```python
from build123d import *

# Parameters (mm, degrees)
BOSS_EXTRUDE2_DEPTH = 25
CUT_EXTRUDE1_REACH  = 76.865
SKETCH5_R           = 2.5
CUT_EXTRUDE4_DEPTH  = 51.520709


with BuildPart() as part:
    # Sketch2 → Boss-Extrude2 (new body)
    with BuildSketch(Plane(origin=(0, 0, 0), x_dir=(0, 0, -1), z_dir=(1, 0, 0))):
        with BuildLine():
            Line((0, 0), (59.16515139, 0))
            ThreePointArc((59.16515139, 0), (67.935731583, -14.803844614), (50.738650505, -15.384615385))
            ThreePointArc((50.738650505, -15.384615385), (49.651853624, -14.368825942), (48.21070024, -14))
            Line((48.21070024, -14), (45, -14))
            Line((45, -14), (0, -14))
            Line((0, -14), (0, -6.25))
            Line((0, -6.25), (47.230433128, -6.25))
            ThreePointArc((47.230433128, -6.25), (50.576761962, -7.534884479), (52.203232404, -10.729166667))
            ThreePointArc((52.203232404, -10.729166667), (65.645099511, -12.64769189), (54.705893308, -4.604166667))
            ThreePointArc((54.705893308, -4.604166667), (53.213216965, -5.454829079), (51.520708964, -5.75))
            Line((51.520708964, -5.75), (0, -5.75))
            Line((0, -5.75), (0, 0))
        make_face()
    extrude(amount=BOSS_EXTRUDE2_DEPTH)

    # Sketch5 → Cut-Extrude1 (cut, up to next)
    with BuildSketch(Plane.XZ.offset(14), mode=Mode.PRIVATE) as cut_extrude1_sk1:
        with Locations(Location((12.5, -30.56070024, 0), (0, 0, 270))):
            Circle(SKETCH5_R)
    cut_extrude1_tool1 = extrude(cut_extrude1_sk1.sketch, amount=-CUT_EXTRUDE1_REACH, mode=Mode.PRIVATE) & part.part
    # Sketch5 → Cut-Extrude1 (cut, up to next)
    with BuildSketch(Plane.XZ.offset(14), mode=Mode.PRIVATE) as cut_extrude1_sk2:
        with Locations(Location((12.5, -38.19070024, 0), (0, 0, 270))):
            Circle(SKETCH5_R)
    cut_extrude1_tool2 = extrude(cut_extrude1_sk2.sketch, amount=-CUT_EXTRUDE1_REACH, mode=Mode.PRIVATE) & part.part
    # Sketch5 → Cut-Extrude1 (cut, up to next)
    with BuildSketch(Plane.XZ.offset(14), mode=Mode.PRIVATE) as cut_extrude1_sk3:
        with Locations(Location((12.5, -44.84070024, 0), (0, 0, 270))):
            Circle(SKETCH5_R)
    cut_extrude1_tool3 = extrude(cut_extrude1_sk3.sketch, amount=-CUT_EXTRUDE1_REACH, mode=Mode.PRIVATE) & part.part
    add(cut_extrude1_tool1.solids().sort_by_distance((12.5, -14, -30.5607))[0], mode=Mode.SUBTRACT)
    add(cut_extrude1_tool2.solids().sort_by_distance((12.5, -14, -38.1907))[0], mode=Mode.SUBTRACT)
    add(cut_extrude1_tool3.solids().sort_by_distance((12.5, -14, -44.8407))[0], mode=Mode.SUBTRACT)

    # Sketch7 → Cut-Extrude4 (cut)
    with BuildSketch(Plane.XY):
        with BuildLine():
            Line((22.5, -6.25), (22.5, -5.75))
            ThreePointArc((22.5, -5.75), (12.5, -2), (2.5, -5.75))
            Line((2.5, -5.75), (2.5, -6.25))
            ThreePointArc((2.5, -6.25), (12.5, -10), (22.5, -6.25))
        make_face()
    extrude(amount=-CUT_EXTRUDE4_DEPTH, mode=Mode.SUBTRACT)


solid = part.part
```
Work out the finished part from the listing and answer in its coordinate system (mm). A direction names the side the tool comes from. Give positions to 0.01 mm unless a question says otherwise; leave off trailing zeros. Write each loop counter-clockwise with the first axis right and the second up, starting at its lowest first coordinate (ties: lowest second). Pieces come first, ordered by that corner, then holes.
(1) Which of the six approach directions +Z, -Z, +X, -X, +Y, -Y give full straight-line access (tool end or side, diameter ignored) to faces 5 (the cylindrical face through (12.325, -5.447, -53.236)), 6 (the cylindrical face through (10.979, -11.926, -42.857)), 7 (the flat face through (24, -6.25, -23)), 8 (the flat face through (12, -9, -51.521))?
Final values:
face 5: +X, -X
face 6: -Y
face 7: +Z, +X, -X
face 8: +Z
(2) The part is cut by section D-D on x = 17. Write down the section's boundary in (y, z).
Final values:
outline: (-15.38, -50.74) arc R10 ccw (long way) to (0, -59.17) - (0, 0) - (-2.68, 0) - (-2.68, -51.52) - (-5.75, -51.52) arc R5 ccw to (-4.6, -54.71) arc R7 cw (long way) to (-10.73, -52.2) arc R5 ccw to (-8.68, -51.52) - (-9.32, -51.52) - (-9.32, 0) - (-14, 0) - (-14, -48.21) arc R3 cw to start
(3) The part is cut by section A-A on z = -21. Write down the section's boundary in (x, y).
Final values:
outline: (0, -14) - (25, -14) - (25, -6.25) - (22.5, -6.25) arc R15.21 cw to (2.5, -6.25) - (0, -6.25) - close; (0, -5.75) - (2.5, -5.75) arc R15.21 cw to (22.5, -5.75) - (25, -5.75) - (25, 0) - (0, 0) - close
(4) The mould has two halves that part along Y. Classify faces 1 (the flat face through (12, -14, -24)), 2 (the cylindrical face through (12.32, -9.49, -51.91)), 3 (the flat face through (12.3, -1.6, 0)), 4 (the cylindrical face through (12.32, -14.55, -68.07)): pulls with the +Y half, pulls with the -Y half, needs draft (parallel to the pull), parting line crosses it, or undercut.
Final values:
face 1: pulls with the -Y half
face 2: undercut
face 3: needs draft
face 4: parting line crosses it
(5) Flat-ended cylindrical pins translate along their axes: pin 1 Ø1.2 at (x, z) = (23, -35) entering from -Y; pin 2 Ø8 at (x, y) = (7, -4) entering from -Z; pin 3 Ø1.5 at (x, y) = (7.5, -6.5) entering from -Z. Find the tip coordinate at first contact, or state that the pin passes through.
Final values:
pin 1: stops at y = -14
pin 2: stops at z = -68.96
pin 3: stops at z = -68.78
(6) The part is cut by section C-C on z = -45. Write down the section's boundary in (x, y), plus the area to 3 significant figures.
Final values:
outline: (0, -14) - (10.01, -14) - (10.01, -9.79) arc R15.21 cw to (2.5, -6.25) - (0, -6.25) - close; (0, -5.75) - (2.5, -5.75) arc R15.21 cw to (22.5, -5.75) - (25, -5.75) - (25, 0) - (0, 0) - close; (14.99, -14) - (25, -14) - (25, -6.25) - (22.5, -6.25) arc R15.21 cw to (14.99, -9.79) - close
area: 214 mm2
(7) The part is cut by section B-B on x = 12.5. Write down the section's boundary in (y, z), plus the area to 3 significant figures.
Final values:
outline: (-15.38, -50.74) arc R10 ccw (long way) to (0, -59.17) - (0, 0) - (-2, 0) - (-2, -51.52) - (-5.75, -51.52) arc R5 ccw to (-4.6, -54.71) arc R7 cw (long way) to (-10.73, -52.2) arc R5 ccw to (-8.68, -51.52) - (-10, -51.52) - (-10, -47.34) - (-14, -47.34) - (-14, -48.21) arc R3 cw to start; (-14, -42.34) - (-10, -42.34) - (-10, -40.69) - (-14, -40.69) - close; (-14, -35.69) - (-10, -35.69) - (-10, -33.06) - (-14, -33.06) - close; (-14, -28.06) - (-10, -28.06) - (-10, 0) - (-14, 0) - close
area: 395 mm2
(8) Straight lines are drawn through the part: line 1 (Y direction, x = 6, z = -59); line 2 (Y direction, x = 13, z = -22); line 3 (Z direction, x = 12.5, y = -11.5). For each, find the intervals that lie inside material, in ascending order.
Final values:
line 1: y = -20 to -17, -3 to 0
line 2: y = -14 to -9.99, -2.01 to 0
line 3: z = -69.05 to -66, -52.33 to -47.34, -42.34 to -40.69, -35.69 to -33.06, -28.06 to 0
